from build123d import *

# Parameters (mm, degrees)
F0_W       = 25.4
F0_H       = 25.4
F1_DEPTH   = 25.4
F2_R       = 2.54
F3_DEPTH   = 17.78
F4_W       = 20.32
F4_H       = 20.32
F5_DEPTH   = 3.81
F6_R       = 2.54
F7_DEPTH   = 1.27
F8_R       = 2.54
F9_DEPTH   = 1.27
F10_R      = 2.54
F1_FACE3_W = 20.32
F1_FACE3_H = 20.32
F11_DEPTH  = 1.27
F12_R      = 2.4632205566
F12_R_2    = 2.54
F13_DEPTH  = 1.27
F14_R      = 2.54
F15_DEPTH  = 1.27
F16_R      = 2.54
F17_DEPTH  = 1.27


with BuildPart() as f1:
    # F0 (on Front) → F1 (new body)
    with BuildSketch(Plane.XZ):
        Rectangle(F0_W, F0_H)
    extrude(amount=F1_DEPTH)

    # F2
    f2_edges = [f1.edges().sort_by_distance(p)[0] for p in [
        (12.7, -12.7, 12.7),
        (12.7, -25.4, 0),
        (12.7, -12.7, -12.7),
        (12.7, 0, 0),
        (0, 0, 12.7),
        (0, 0, -12.7),
        (0, -25.4, -12.7),
        (0, -25.4, 12.7),
        (-12.7, -25.4, 0),
        (-12.7, -12.7, 12.7),
        (-12.7, 0, 0),
        (-12.7, -12.7, -12.7),
    ]]
    fillet(f2_edges, radius=F2_R)

    # F3 (cut): a face of the model
    f3_faces = [f1.faces().sort_by_distance(p)[0] for p in [
        (0, 0, 0),
    ]]
    extrude(f3_faces, amount=-F3_DEPTH, mode=Mode.SUBTRACT)

    # F4 (on Front) → F5 (join)
    with BuildSketch(Plane.XZ):
        Rectangle(F4_W, F4_H)
    extrude(amount=F5_DEPTH)

    # F6 (on face) → F7 (cut)
    with BuildSketch(Plane(origin=(0, 0, 0), x_dir=(-1, 0, 0), z_dir=(0, 1, 0))):
        with Locations((-5.6349025984, 0)):
            Circle(F6_R)
        with Locations((-5.6349025984, 6.9014462642)):
            Circle(F6_R)
        with Locations((-5.6349025984, -5.9648556635)):
            Circle(F6_R)
        with Locations((5.1562977023, 0)):
            Circle(F6_R)
        with Locations((5.1562977023, 6.9774198346)):
            Circle(F6_R)
        with Locations((5.1562977023, -6.0284850188)):
            Circle(F6_R)
    extrude(amount=-F7_DEPTH, mode=Mode.SUBTRACT)

    # F8 (on face) → F9 (cut)
    with BuildSketch(Plane.XZ.offset(25.4)):
        Circle(F8_R)
    extrude(amount=-F9_DEPTH, mode=Mode.SUBTRACT)

    # F10 (on face) + F1_face3 (on face) → F11 (cut)
    with BuildSketch(Plane.YZ.offset(12.7)):
        with Locations((-12.7, 0)):
            Circle(F10_R)
        with Locations((-6.582416594, 6.4226952381)):
            Circle(F10_R)
        with Locations((-19.1999990493, -6.0931327753)):
            Circle(F10_R)
    with BuildSketch(Plane(origin=(-12.7, -12.7, 0), x_dir=(0, -1, 0), z_dir=(-1, 0, 0))):
        Rectangle(F1_FACE3_W, F1_FACE3_H)
    extrude(amount=-F11_DEPTH, dir=(1, 0, 0), mode=Mode.SUBTRACT)

    # F12 (on face) → F13 (cut)
    with BuildSketch(Plane(origin=(-12.7, 0, 0), x_dir=(0, -1, 0), z_dir=(-1, 0, 0))):
        with Locations((6.9892560132, 6.1440924183)):
            Circle(F12_R)
        with Locations((6.9892560132, -5.2524344064)):
            Circle(F12_R_2)
        with Locations((18.284028396, 6.1440924183)):
            Circle(F12_R_2)
        with Locations((18.284028396, -5.2524344064)):
            Circle(F12_R_2)
    extrude(amount=-F13_DEPTH, mode=Mode.SUBTRACT)

    # F14 (on face) → F15 (cut)
    with BuildSketch(Plane(origin=(0, 0, -12.7), x_dir=(1, 0, 0), z_dir=(0, 0, -1))):
        with Locations((4.888321273, 18.5727626085)):
            Circle(F14_R)
        with Locations((-4.9818856642, 8.193783462)):
            Circle(F14_R)
    extrude(amount=-F15_DEPTH, mode=Mode.SUBTRACT)

    # F16 (on face) → F17 (cut)
    with BuildSketch(Plane.XY.offset(12.7)):
        with Locations((0, -11.8432976305)):
            Circle(F16_R)
        with Locations((-6.1014243402, -6.1122667976)):
            Circle(F16_R)
        with Locations((6.108049769, -6.1122667976)):
            Circle(F16_R)
        with Locations((-6.1014243402, -19.2499253899)):
            Circle(F16_R)
        with Locations((6.108049769, -19.2499253899)):
            Circle(F16_R)
    extrude(amount=-F17_DEPTH, mode=Mode.SUBTRACT)


solid = f1.part
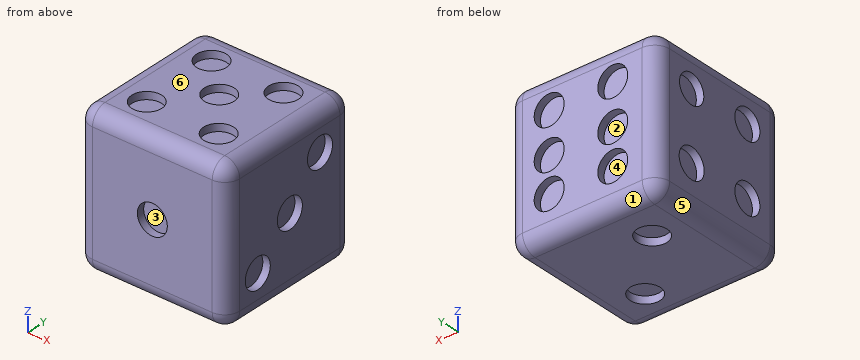
The model under review builds one solid part; all positions refer to its coordinate system, in mm. Face numbers are marked on the shaded views. A direction names the side the tool comes from. Coordinates: 2 decimals unless noted, no trailing zeros. Loops run counter-clockwise (first coordinate to the right, second up) from the corner with the lowest first, then second, coordinate; pieces in that order, holes last. Notation, with made-up numbers: M 78.25,-29 L 103.25,-29 A6 ccw 103.25,-18 Z; hole C -9,75 d6. An arc over 180 degrees is marked long. Put each result on its own line as item: value. Start each with the question number.
Q1. Wall thickness on line 1 (Y direction, x = -7.75, z = 3.25); line 2 (Y direction, x = 7.25, z = -0.25); line 3 (Z direction, x = -7, y = -5.25): over which ranges is each line inside the solid? List them lowest first.
Q2. The part is to be moulded in two halves that separate along X. For the marked faces 4, 5 and 6, say which applies: +X half, -X half, draft (parallel to the pull), parting line (faces both ways), or undercut.
Q3. Add section A-A (z = 0). Write out the cut boundary in (x, y).
Q4. For the marked faces 1, 2 and 3, list the 3-axis set-ups (+Z, -Z, +X, -X, +Y, -Y) from which the entire face can be reached by the end or side of a thin tool; tool diameter is ignored.
Q5. Clearance check with a flat-ended pin moving along its axis: pin 1 (4.5 mm diameter, centred on x = 6.11, y = -19.25, fed in from +Z). State where the tip first meets the part, or that it passes through.
Q6. Add section D-D (y = -12.7). Write out the cut boundary in (x, z), and give its area (3 significant figures).
Q7. Add section B-B (x = 0). Write out the cut boundary in (y, z), and give its area (3 significant figures).
Answers:
1. line 1: y = -25.4 to -17.78, -3.81 to 0
1. line 2: y = -25.4 to -17.78, -3.81 to -1.27
1. line 3: z = -12.7 to -10.16, 10.16 to 11.43
2. face 4: undercut
2. face 5: -X half
2. face 6: draft
3. outline: M -12.7,-22.86 A2.54 ccw -10.16,-25.4 L -2.54,-25.4 L -2.54,-24.13 L 2.54,-24.13 L 2.54,-25.4 L 10.16,-25.4 A2.54 ccw 12.7,-22.86 L 12.7,-15.24 L 11.43,-15.24 L 11.43,-10.16 L 12.7,-10.16 L 12.7,-2.54 A2.54 ccw 10.16,0 L 8.17,0 L 8.17,-1.27 L 3.09,-1.27 L 3.09,0 L -2.62,0 L -2.62,-1.27 L -7.7,-1.27 L -7.7,0 L -10.16,0 A2.54 ccw -12.7,-2.54 Z; hole M -10.16,-17.78 L 10.16,-17.78 L 10.16,-3.81 L -10.16,-3.81 Z
4. face 1: -Z, +X, -X, +Y
4. face 2: +Y
4. face 3: -Y
5. pin 1: stops at z = 11.43
6. outline: M -12.7,-10.16 A2.54 ccw -10.16,-12.7 L 10.16,-12.7 A2.54 ccw 12.7,-10.16 L 12.7,-2.54 L 11.43,-2.54 L 11.43,2.54 L 12.7,2.54 L 12.7,10.16 A2.54 ccw 10.16,12.7 L 2.39,12.7 L 2.39,11.43 L -2.39,11.43 L -2.39,12.7 L -10.16,12.7 A2.54 ccw -12.7,10.16 Z; hole M -10.16,-10.16 L 10.16,-10.16 L 10.16,10.16 L -10.16,10.16 Z
6. area: 214 mm^2
7. outline: M -25.4,-10.16 A2.54 ccw -22.86,-12.7 L -2.54,-12.7 A2.54 ccw 0,-10.16 L 0,10.16 A2.54 ccw -2.54,12.7 L -9.3,12.7 L -9.3,11.43 L -14.38,11.43 L -14.38,12.7 L -22.86,12.7 A2.54 ccw -25.4,10.16 L -25.4,2.54 L -24.13,2.54 L -24.13,-2.54 L -25.4,-2.54 Z; hole M -17.78,-10.16 L -3.81,-10.16 L -3.81,10.16 L -17.78,10.16 Z
7. area: 343 mm^2
